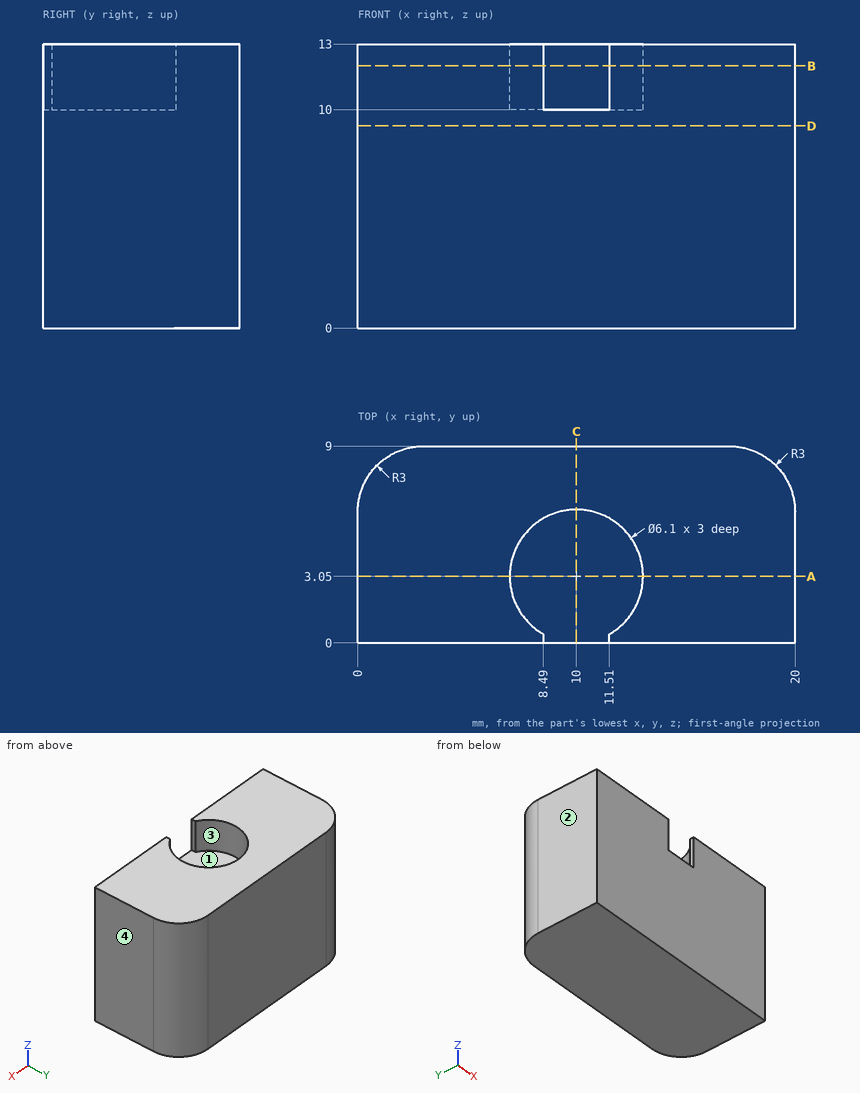
Geometry check sheet. Reference: drawing and pictorial views, mm from the part's lowest x, y, z. Coordinates: 2 decimals unless noted, no trailing zeros. Write each loop counter-clockwise with the first axis right and the second up, starting at its lowest first coordinate (ties: lowest second). Pieces come first, ordered by that corner, then holes. Notation, with made-up numbers: (16.5, 48) - (33.5, 48) arc R17 cw to (33.5, 71) - close; hole circle Ø4 at (67, -5). An arc over 180 degrees is marked (long way). One line per question, with ' | ' between items. Start each with the question number.
1. Material ranges on line 1 along X through (y, z) = (3.05, 11); line 2 along Y through (x, z) = (10, 12.05); line 3 along Z through (x, y) = (10.25, 5.25), recorded low to high.
2. Section check A-A (y = 3.05). Enter the section's corners in (x, z).
3. Section check B-B (z = 12). Enter the section's corners in (x, y), plus the area to 3 significant figures.
4. Draft check along X on the marked faces 1, 2, 3 and 4. Enter one of: released by +X, released by -X, zero draft, split by the parting line, or undercut.
5. Section check D-D (z = 9.25). Enter the section's corners in (x, y).
6. Gauge pin test, flat ends, axial feed: P1, Ø5, axis at x = 10, y = 3.05, coming from the +Z side; P2, Ø1, axis at y = 7, z = 8, coming from the +X side. Record the tip position at first contact, or that the pin passes through.
7. Section check C-C (x = 10). Enter the section's corners in (y, z).
Computed values:
1) line 1: 0 to 6.95, 13.05 to 20 | line 2: 6.1 to 9 | line 3: 0 to 10
2) outline: (0, 0) - (20, 0) - (20, 13) - (13.05, 13) - (13.05, 10) - (6.95, 10) - (6.95, 13) - (0, 13) - close
3) outline: (0, 0) - (8.49, 0) - (8.49, 0.4) arc R3.05 cw (long way) to (11.51, 0.4) - (11.51, 0) - (20, 0) - (20, 6) arc R3 ccw to (17, 9) - (3, 9) arc R3 ccw to (0, 6) - close | area: 147 mm²
4) face 1: undercut | face 2: released by -X | face 3: undercut | face 4: released by +X
5) outline: (0, 0) - (20, 0) - (20, 6) arc R3 ccw to (17, 9) - (3, 9) arc R3 ccw to (0, 6) - close
6) P1: z = 10 | P2: x = 19.96
7) outline: (0, 0) - (9, 0) - (9, 13) - (6.1, 13) - (6.1, 10) - (0, 10) - close
